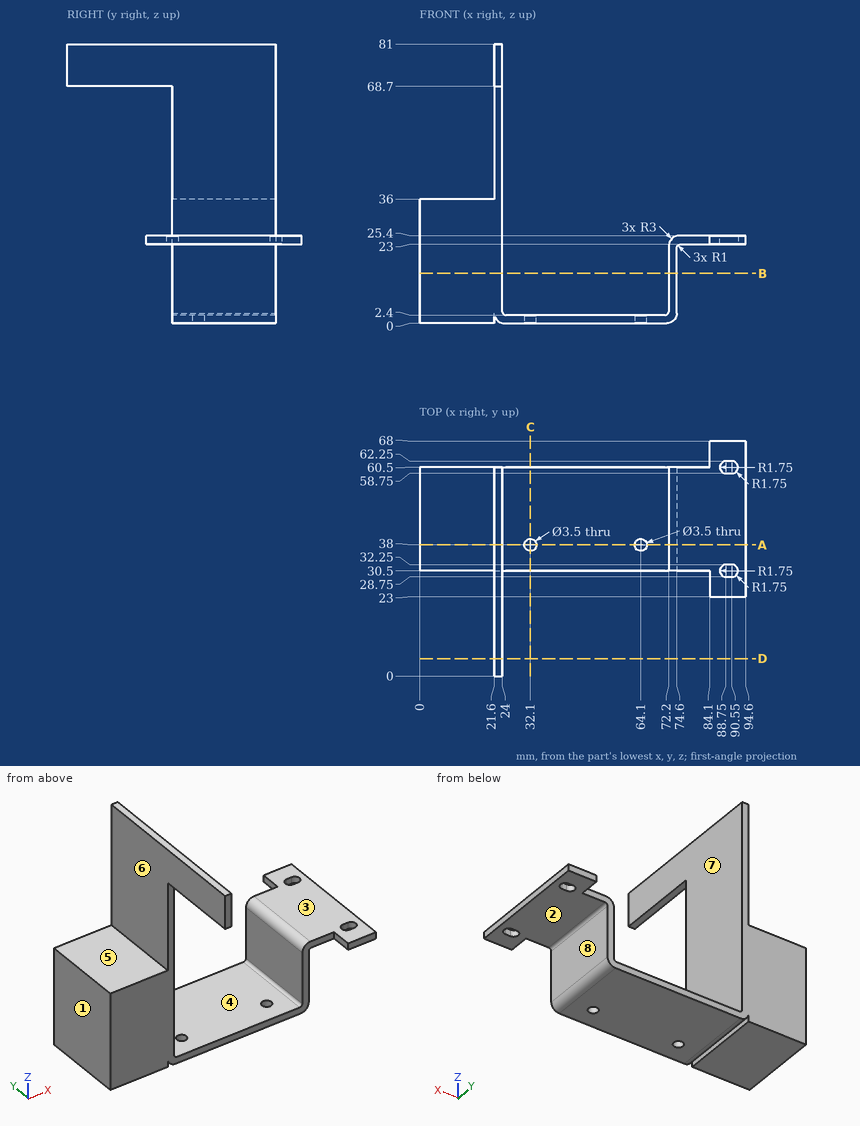
Drawing for the job (mm, zero at the part's lowest x, y, z). A direction names the side the tool comes from. Give positions to 0.01 mm unless a question says otherwise; leave off trailing zeros. Loops run counter-clockwise (first coordinate to the right, second up) from the corner with the lowest first, then second, coordinate; pieces in that order, holes last. Notation, with made-up numbers: M 65.25,82.5 L 93.25,82.5 A4 ccw 93.25,89.5 Z; hole C 40.25,17.5 d10. An arc over 180 degrees is marked long. Use one line per item in the form item = value.
Item 1: Slice it at B-B (z = 14.5). List the corners of the cut face in (x, y).
Determined:
outline = M 0,30.5 L 24,30.5 L 24,60.5 L 0,60.5 Z; M 72.2,30.5 L 74.6,30.5 L 74.6,60.5 L 72.2,60.5 Z
Item 2: Slice it at D-D (y = 5). List the corners of the cut face in (x, z), plus the area to 3 significant figures.
Determined:
outline = M 21.6,68.7 L 24,68.7 L 24,81 L 21.6,81 Z
area = 29.5 mm2
Item 3: Slice it at C-C (x = 32.1). List the corners of the cut face in (y, z).
Determined:
outline = M 30.5,0 L 36.25,0 L 36.25,2.4 L 30.5,2.4 Z; M 39.75,0 L 60.5,0 L 60.5,2.4 L 39.75,2.4 Z
Item 4: Flat gauge pins, fed straight in: pin 1 (2 mm diameter, centred on x = 49.5, y = 52.5, fed in from +Z); pin 2 (1.2 mm diameter, centred on x = 87.5, z = 23.5, fed in from -Y); pin 3 (5 mm diameter, centred on x = 71.5, z = 19, fed in from +Y). Where does each tip first touch, or does it go through?
Determined:
pin_1 = 2.4
pin_2 = 23
pin_3 = 60.5
Item 5: Slice it at A-A (y = 38). List the corners of the cut face in (x, z).
Determined:
outline = M 0,0 L 21.6,0 L 21.6,3 A3 ccw 24.6,0 L 30.35,0 L 30.35,2.4 L 25,2.4 A1 cw 24,3.4 L 24,81 L 21.6,81 L 21.6,36 L 0,36 Z; M 33.85,0 L 62.35,0 L 62.35,2.4 L 33.85,2.4 Z; M 65.85,0 L 71.6,0 A3 ccw 74.6,3 L 74.6,22 A1 cw 75.6,23 L 94.6,23 L 94.6,25.4 L 75.2,25.4 A3 ccw 72.2,22.4 L 72.2,3.4 A1 cw 71.2,2.4 L 65.85,2.4 Z
Item 6: Two-plate mould, pull along X, no slides. Class the marked faces 6, 7 and 8: pulls with the +X half, pulls with the -X half, needs draft (parallel to the pull), parting line crosses it, or undercut.
Determined:
face_6 = pulls with the -X half
face_7 = undercut
face_8 = pulls with the +X half
Item 7: Which spindle directions (+Z, -Z, +X, -X, +Y, -Y) get a long thin tool onto all of the face, cutting with end or side? Do the marked faces 1, 2, 3, 4 and 5. Say none if no direction does.
Determined:
face_1 = +Z, -Z, -X, +Y, -Y
face_2 = -Z, +X, +Y, -Y
face_3 = +Z, +X, +Y, -Y
face_4 = +Z, +Y, -Y
face_5 = +Z, -X, +Y, -Y
Item 8: Drill centre lines: probe 1 along Y at (x, z) = (64.1, 1.95); probe 2 along X at (y, z) = (31.5, 16); probe 3 along X at (y, z) = (38, 1.55). Where is each one in solid material? Low to high. Write a range as from..to.
Determined:
probe_1 = 30.5..36.25, 39.75..60.5
probe_2 = 0..24, 72.2..74.6
probe_3 = 0..21.6, 21.97..30.35, 33.85..62.35, 65.85..74.23
